```python
from build123d import *

# Parameters (mm, degrees)
SKETCH1_W           = 150
SKETCH1_H           = 150
BOSS_EXTRUDE1_DEPTH = 10
CHAMFER1_SIZE       = 30
CHAMFER1_SIZE2      = 80
CHAMFER2_SIZE       = 80
CHAMFER2_SIZE2      = 30
SKETCH2_R           = 8
CUT_EXTRUDE1_DEPTH  = 10


with BuildPart() as part:
    # Sketch1 → Boss-Extrude1 (new body)
    with BuildSketch(Plane(origin=(0, 0, 0), x_dir=(1, 0, 0), z_dir=(0, 1, 0))):
        with Locations((75, 75)):
            Rectangle(SKETCH1_W, SKETCH1_H)
    extrude(amount=BOSS_EXTRUDE1_DEPTH)

    # Chamfer1
    chamfer1_edges = [part.edges().sort_by_distance(p)[0] for p in [
        (0, 5, 0),
    ]]
    chamfer1_side = [part.faces().sort_by_distance(p)[0] for p in [
        (0, 5, -75),
    ]]
    chamfer(chamfer1_edges, length=CHAMFER1_SIZE, length2=CHAMFER1_SIZE2, reference=chamfer1_side[0])

    # Chamfer2
    chamfer2_edges = [part.edges().sort_by_distance(p)[0] for p in [
        (0, 5, -150),
    ]]
    chamfer2_side = [part.faces().sort_by_distance(p)[0] for p in [
        (75, 5, -150),
    ]]
    chamfer(chamfer2_edges, length=CHAMFER2_SIZE, length2=CHAMFER2_SIZE2, reference=chamfer2_side[0])

    # Sketch2 → Cut-Extrude1 (cut)
    with BuildSketch(Plane(origin=(0, 10, 0), x_dir=(1, 0, 0), z_dir=(0, 1, 0))):
        with Locations((134, 134)):
            Circle(SKETCH2_R)
        with Locations((134, 16)):
            Circle(SKETCH2_R)
        with Locations((20, 105)):
            Circle(SKETCH2_R)
        with Locations((20, 45)):
            Circle(SKETCH2_R)
    extrude(amount=-CUT_EXTRUDE1_DEPTH, mode=Mode.SUBTRACT)


solid = part.part
```
Design review of the part built by this model. Coordinates are the model's own, in mm. Give positions to 0.01 mm unless a question says otherwise; leave off trailing zeros. Loops run counter-clockwise (first coordinate to the right, second up) from the corner with the lowest first, then second, coordinate; pieces in that order, holes last. Notation, with made-up numbers: M 16,54 L 48,54 A30 cw 48,77 Z; hole C 65,-36 d10. An arc over 180 degrees is marked long. Return JSON: item names as keys, results as strings. Group by question number.
Item 1: We need section C-C (y = 3). Give the boundary of the cut face in (x, z), and give its area (3 significant figures).
Item 2: We need section A-A (x = 20). Give the boundary of the cut face in (y, z).
Item 3: We need section B-B (z = -45). Give the boundary of the cut face in (x, y), and give its area (3 significant figures).
Item 4: Mouldability with a two-part tool opening along X and no side actions: class faces 1 (the flat face through (40.56, 4.93, -14.79)), 2 (the cylindrical face through (137.69, 5.07, -126.9)), 3 (the flat face through (74, 10, -76)) as released by +X, released by -X, zero draft, split by the parting line, or undercut.
Item 5: Insertion check: pin 1 Ø5 at (x, y) = (88, 5.5) entering from +Z. The pin has a flat end and moves straight along its axis. Give the tip position at first contact, or say it passes through.
Item 6: For probe 1 along Z at (x, y) = (134, 5.5); probe 2 along Z at (x, y) = (20, 2.25); probe 3 along Z at (x, y) = (42, 8.75), list the stretches that pass through material, from the lowest coordinate up.
Item 7: We need section D-D (x = 134). Give the boundary of the cut face in (y, z), and give its area (3 significant figures).
Output:
{
 "1": {"outline": "M 0,-120 L 80,-150 L 150,-150 L 150,0 L 80,0 L 0,-30 Z; hole C 20,-105 d16; hole C 20,-45 d16; hole C 134,-134 d16; hole C 134,-16 d16", "area": "19,300 mm^2"},
 "2": {"outline": "M 0,-127.5 L 10,-127.5 L 10,-113 L 0,-113 Z; M 0,-97 L 10,-97 L 10,-53 L 0,-53 Z; M 0,-37 L 10,-37 L 10,-22.5 L 0,-22.5 Z"},
 "3": {"outline": "M 0,0 L 12,0 L 12,10 L 0,10 Z; M 28,0 L 150,0 L 150,10 L 28,10 Z", "area": "1,340 mm^2"},
 "4": {"face 1": "released by -X", "face 2": "undercut", "face 3": "zero draft"},
 "5": {"pin 1": "stops at z = 0"},
 "6": {"probe 1": "z = -150 to -142, -126 to -24, -8 to 0", "probe 2": "z = -127.5 to -113, -97 to -53, -37 to -22.5", "probe 3": "z = -135.75 to -14.25"},
 "7": {"outline": "M 0,-150 L 10,-150 L 10,-142 L 0,-142 Z; M 0,-126 L 10,-126 L 10,-24 L 0,-24 Z; M 0,-8 L 10,-8 L 10,0 L 0,0 Z", "area": "1,180 mm^2"}
}
